```python
from build123d import *

# Parameters (mm, degrees)
SZKIC1_W                    = 15
SZKIC1_H                    = 40
DODANIE_WYCI_GNI_CIE1_DEPTH = 5
SZKIC2_W                    = 10
SZKIC2_H                    = 10
DODANIE_WYCI_GNI_CIE2_DEPTH = 10
SZKIC3_R                    = 4
WYTNIJ_WYCI_GNI_CIE1_DEPTH  = 30
ZAOKR_GLENIE1_R             = 5
SZKIC4_R                    = 4
WYTNIJ_WYCI_GNI_CIE2_DEPTH  = 30


with BuildPart() as part:
    # Szkic1 → Dodanie-wyciągnięcie1 (new body)
    with BuildSketch(Plane(origin=(0, 0, 0), x_dir=(1, 0, 0), z_dir=(0, 1, 0))):
        Rectangle(SZKIC1_W, SZKIC1_H)
    extrude(amount=DODANIE_WYCI_GNI_CIE1_DEPTH)

    # Szkic2 → Dodanie-wyciągnięcie2 (add)
    with BuildSketch(Plane(origin=(7.5, 0, 0), x_dir=(0, 0, -1), z_dir=(1, 0, 0))):
        with Locations((-15, 5)):
            Rectangle(SZKIC2_W, SZKIC2_H)
        with Locations((5, 5)):
            Rectangle(SZKIC2_W, SZKIC2_H)
    extrude(amount=DODANIE_WYCI_GNI_CIE2_DEPTH)

    # Szkic3 → Wytnij-wyciągnięcie1 (cut)
    with BuildSketch(Plane.XY.offset(20)):
        with Locations((12.5, 5)):
            Circle(SZKIC3_R)
    extrude(amount=-WYTNIJ_WYCI_GNI_CIE1_DEPTH, mode=Mode.SUBTRACT)

    # Zaokrąglenie1
    zaokr_glenie1_edges = [part.edges().sort_by_distance(p)[0] for p in [
        (7.5, 10, 15),
        (7.5, 10, -5),
        (17.5, 0, 15),
        (17.5, 0, -5),
        (17.5, 10, -5),
        (17.5, 10, 15),
    ]]
    fillet(zaokr_glenie1_edges, radius=ZAOKR_GLENIE1_R - 0.0001)  # a hair under: the kernel refuses the full size

    # Szkic4 → Wytnij-wyciągnięcie2 (cut)
    with BuildSketch(Plane(origin=(0, 5, 0), x_dir=(1, 0, 0), z_dir=(0, 1, 0))):
        with Locations(Location((0, 10, 0), (0, 0, 270))):
            Circle(SZKIC4_R)
        with Locations(Location((0, -10, 0), (0, 0, 270))):
            Circle(SZKIC4_R)
    extrude(amount=-WYTNIJ_WYCI_GNI_CIE2_DEPTH, mode=Mode.SUBTRACT)


solid = part.part
```
Verification items for the finished model (mm, model axes). A direction names the side the tool comes from. Give positions to 0.01 mm unless a question says otherwise; leave off trailing zeros. Loops run counter-clockwise (first coordinate to the right, second up) from the corner with the lowest first, then second, coordinate; pieces in that order, holes last. Notation, with made-up numbers: M 17.5,16 L 38.5,16 A11 ccw 38.5,26 Z; hole C -28,79.25 d2. An arc over 180 degrees is marked long. One line per question, with ' | ' between items.
Item 1: Section check B-B, the plane y = 1.5. Record the cut outline in (x, z), plus the area to 3 significant figures.
Completed:
outline: M -7.5,-20 L 7.5,-20 L 7.5,-10 L 10.56,-10 L 10.56,0 L 7.5,0 L 7.5,10 L 10.56,10 L 10.56,20 L -7.5,20 Z; M 14.44,-10 L 16.07,-10 L 16.07,0 L 14.44,0 Z; M 14.44,10 L 16.07,10 L 16.07,20 L 14.44,20 Z; hole C 0,-10 d8; hole C 0,10 d8 | area: 593 mm^2
Item 2: Draft check along X on faces 4 (the face through (-7.5, 2, 0)), 5 (the face through (9.3, 2.6, 15.1)), 6 (the face through (0, 5, 0)). Enter one of: +X half, -X half, draft (parallel to the pull), parting line (faces both ways), or undercut.
Completed:
face 4: -X half | face 5: undercut | face 6: draft
Item 3: Section check A-A, the plane x = 0. Record the cut outline in (y, z), plus the area to 3 significant figures.
Completed:
outline: M 0,-20 L 5,-20 L 5,-14 L 0,-14 Z; M 0,-6 L 5,-6 L 5,6 L 0,6 Z; M 0,14 L 5,14 L 5,20 L 0,20 Z | area: 120 mm^2
Item 4: Section check D-D, the plane z = -11.5. Record the cut outline in (x, y).
Completed:
outline: M -7.5,0 L -3.71,0 L -3.71,5 L -7.5,5 Z; M 3.71,0 L 7.5,0 L 7.5,5 L 3.71,5 Z
Item 5: Tool access check on faces 1 (the face through (5, 3, 20)), 2 (the face through (11, 1, 10)), 3 (the face through (11, 1, -10)). Record the directions out of +Z, -Z, +X, -X, +Y, -Y that give a thin tool (end or side, any length) a straight path to the whole face; none if there is none.
Completed:
face 1: +Z, +X, -X, +Y, -Y | face 2: +X, +Y, -Y | face 3: -Z, +X, +Y, -Y
Item 6: Depth check by flat-ended pin: P1, Ø5, axis at x = 1, z = 4, coming from the +Y side; P2, Ø1.5, axis at y = 3.5, z = 4, coming from the +X side; P3, Ø9, axis at x = 0, z = 10, coming from the -Y side. Enter the tip coordinate at first touch or a pass-through.
Completed:
P1: stops at y = 5 | P2: stops at x = 7.5 | P3: stops at y = 0
Item 7: Thickness scan on line 1 (Z direction, x = 8.75, y = 8); line 2 (Z direction, x = -3.25, y = 0.5); line 3 (Z direction, x = -3, y = 2.25). Record the ranges inside material, lowest first. Write a range as [from, to].
Completed:
line 1: z = [-10, 0], [10, 20] | line 2: z = [-20, -12.33], [-7.67, 7.67], [12.33, 20] | line 3: z = [-20, -12.65], [-7.35, 7.35], [12.65, 20]
